Input: part model. Units: mm. Frame: model coordinates. A direction names the side the tool comes from. Round coordinates to 2 decimals unless told otherwise and drop trailing zeros. Loops run counter-clockwise (first coordinate to the right, second up) from the corner with the lowest first, then second, coordinate; pieces in that order, holes last. Notation, with made-up numbers: (20, -7) - (47, -7) arc R27 cw to (47, 30) - close; hole circle Ø8 at (55, 35.25). An arc over 180 degrees is marked (long way). One line per question, with ' | ' between items. Start each with the question number.
Item 1: Draft query along Y for faces 4 (the face through (3, 40.945, 13)), 5 (the face through (-26, -25, 25.4)), 6 (the face through (10.58, 34.005, 24.293)). Return one class per face: pulls with the +Y half, pulls with the -Y half, needs draft (parallel to the pull), parting line crosses it, or undercut.
Item 2: Section C-C, the plane z = 30.5. Return loops of the section in (x, y), plus the area to 3 significant figures.
Item 3: First-contact query: pin 1 (4 mm diameter, centred on x = -23, z = 29.5, fed in from -Y); pin 2 (8 mm diameter, centred on y = -36, z = 39, fed in from +X); pin 3 (7 mm diameter, centred on y = 12, z = 41.5, fed in from -X); pin 4 (24 mm diameter, centred on x = 3.43, y = 22.78, fed in from -Z). Flat tips, straight axial feed; report the tip coordinate or a pass-through.
Item 4: Material intervals for line 1 along Y through (x, z) = (-6.5, 2); line 2 along Y through (x, z) = (-1, 16); line 3 along Z through (x, y) = (13, -8), sorted ascending.
Item 5: Section A-A, the plane x = 0. Give the number of separate pieces and of enclosed holes in the cut face, plus the area to 3 significant figures.
Item 6: Section B-B, the plane y = -41. Return loops of the section in (x, z), plus the area to 3 significant figures.
Item 7: Set-up query: faces 1 (the face through (-25.014, 20, 37)), 2 (the face through (4, -56.369, 31)), 3 (the face through (32.552, -14, 31)). Return all of +Z, -Z, +X, -X, +Y, -Y with unobstructed straight access to the full face (end or side cutting, diameter ignored); none if empty.
```python
from build123d import *

# Parameters (mm, degrees)
F0_W     = 78.810706
F0_H     = 107.936401
F1_DEPTH = 25.4
F2_W     = 57.223428
F2_H     = 86.349123
F3_DEPTH = 37.084
F4_W     = 57.223426
F4_H     = 40.945355
F5_DEPTH = 49.276
F6_R     = 13.306324
F8_DEPTH = 92.456
F7_R     = 16.734073
F9_DEPTH = 76.962


with BuildPart() as f1:
    # F0 (on Top) → F1 (new body)
    with BuildSketch(Plane.XY):
        with Locations((3.083896, -13.022845)):
            Rectangle(F0_W, F0_H)
    extrude(amount=F1_DEPTH)

    # F2 (on Top) → F3 (join)
    with BuildSketch(Plane.XY):
        with Locations((3.940536, -13.194174)):
            Rectangle(F2_W, F2_H)
    extrude(amount=F3_DEPTH)

    # F4 (on Top) → F5 (join)
    with BuildSketch(Plane.XY):
        with Locations((3.597881, 20.472677)):
            Rectangle(F4_W, F4_H)
    extrude(amount=F5_DEPTH)

    # F6 (on Top) → F8 (cut)
    with BuildSketch(Plane.XY):
        with Locations((3.426551, 22.784626)):
            Circle(F6_R)
    extrude(amount=F8_DEPTH, mode=Mode.SUBTRACT)

    # F7 (on Top) → F9 (cut)
    with BuildSketch(Plane.XY):
        with Locations((3.769206, -28.956316)):
            Circle(F7_R)
    extrude(amount=F9_DEPTH, mode=Mode.SUBTRACT)


solid = f1.part
```
Return value:
1) face 4: pulls with the +Y half | face 5: needs draft | face 6: undercut
2) outline: (-25.01, 0) - (-24.67, 0) - (-24.67, -56.37) - (32.55, -56.37) - (32.55, 29.98) - (32.21, 29.98) - (32.21, 40.95) - (-25.01, 40.95) - close; hole circle Ø33.47 at (3.77, -28.96); hole circle Ø26.61 at (3.43, 22.78) | area: 4,140 mm2
3) pin 1: y = -56.37 | pin 2: x = 32.55 | pin 3: x = -25.01 | pin 4: through
4) line 1: -66.99 to -42.17, -15.74 to 13.92, 31.65 to 40.95 | line 2: -66.99 to -45, -12.92 to 10.24, 35.33 to 40.95 | line 3: 0 to 37.08
5) separate pieces: 3 | enclosed holes: 0 | area: 1,900 mm2
6) outline: (-36.32, 0) - (-7.85, 0) - (-7.85, 37.08) - (-24.67, 37.08) - (-24.67, 25.4) - (-36.32, 25.4) - close; (15.39, 0) - (42.49, 0) - (42.49, 25.4) - (32.55, 25.4) - (32.55, 37.08) - (15.39, 37.08) - close | area: 1,810 mm2
7) face 1: +Z, -X, +Y, -Y | face 2: +Z, +X, -X, -Y | face 3: +Z, +X, +Y, -Y
